Work out the finished part from the listing and answer in its coordinate system (mm). Face numbers are marked on the shaded views. A direction names the side the tool comes from. Round coordinates to 2 decimals unless told otherwise and drop trailing zeros. Order: outer loops, then holes, each group sorted by start corner. A loop starts at its lowest first (then second) coordinate and runs counter-clockwise, first axis right, second up. Notation, with made-up numbers: (-36.5, 58.25) -> (19.5, 58.25) arc R32 cw to (19.5, 89.25) -> close; hole circle Ø5 at (-5, 19). An arc over 180 degrees is marked (long way). Use one line per item in the form item = value.
```python
from build123d import *

# Parameters (mm, degrees)
SALIENTE_EXTRUIR1_DEPTH = 51.5
CORTAR_EXTRUIR2_DEPTH   = 25.75
CROQUIS5_R              = 4.05
CROQUIS5_R_2            = 1.6
CORTAR_EXTRUIR3_DEPTH   = 108.820452605
REDONDEO1_R             = 10
REDONDEO2_R             = 2
REDONDEO3_R             = 2


with BuildPart() as part:
    # Croquis1 → Saliente-Extruir1 (new body)
    with BuildSketch(Plane(origin=(0, 0, 0), x_dir=(1, 0, 0), z_dir=(0, 1, 0))):
        with BuildLine():
            Line((75, -12.5), (-58.334166688, -12.5))
            ThreePointArc((-58.334166688, -12.5), (-61.46808254, -13.003760143), (-64.286250013, -14.464285714))
            ThreePointArc((-64.286250013, -14.464285714), (-93, 0), (-64.286250013, 14.464285714))
            ThreePointArc((-64.286250013, 14.464285714), (-61.46808254, 13.003760143), (-58.334166688, 12.5))
            Line((-58.334166688, 12.5), (75, 12.5))
            ThreePointArc((75, 12.5), (87.5, 0), (75, -12.5))
        make_face()
    extrude(amount=SALIENTE_EXTRUIR1_DEPTH)

    # Croquis3 → Cortar-Extruir2 (cut, symmetric)
    with BuildSketch(Plane.XY):
        Polygon((87.5, 25), (-5, 25), (-31.5, 51.5), (87.5, 51.5), align=None)
        Polygon((-15.355339059, 0), (-41.855339059, 26.5), (-93, 26.5), (-93, 0), align=None)
    extrude(amount=CORTAR_EXTRUIR2_DEPTH, both=True, mode=Mode.SUBTRACT)

    # Croquis4 → Cortar-Revoluci_n1 (revolve, cut)
    with BuildSketch(Plane.XY, mode=Mode.PRIVATE) as cortar_revoluci_n1_sk:
        Polygon((-75, 26.5), (-75, 51.5), (-85, 51.5), (-85, 42.5), (-91.1, 35.5), (-91.1, 26.5), align=None)
    revolve(cortar_revoluci_n1_sk.sketch.rotate(Axis((-75, 26.5, 0), (0, 1, 0)), 270), axis=Axis((-75, 26.5, 0), (0, 1, 0)), mode=Mode.SUBTRACT)

    # Croquis5 → Cortar-Extruir3 (cut, through all)
    with BuildSketch(Plane(origin=(0, 0, 0), x_dir=(1, 0, 0), z_dir=(0, 1, 0))):
        with Locations((75, 0)):
            Circle(CROQUIS5_R)
        with Locations((50, 0)):
            Circle(CROQUIS5_R_2)
    extrude(amount=CORTAR_EXTRUIR3_DEPTH, mode=Mode.SUBTRACT)

    # Redondeo1
    redondeo1_edges = [part.edges().sort_by_distance(p)[0] for p in [
        (-31.5, 51.5, 0),
        (-5, 25, 0),
    ]]
    fillet(redondeo1_edges, radius=REDONDEO1_R)

    # Redondeo2
    redondeo2_edges = [part.edges().sort_by_distance(p)[0] for p in [
        (-61.46808254, 51.5, -13.003760143),
        (-93, 51.5, 0),
        (-61.46808254, 51.5, 13.003760143),
        (-46.988151156, 51.5, 12.5),
        (37.071067812, 25, 12.5),
        (87.5, 25, 0),
        (-18.25, 38.25, 12.5),
        (-18.25, 38.25, -12.5),
        (-31.8153013, 50.738795325, 12.5),
        (-46.988151156, 51.5, -12.5),
        (37.071067812, 25, -12.5),
        (-31.8153013, 50.738795325, -12.5),
        (-4.6846987, 25.761204675, 12.5),
        (-4.6846987, 25.761204675, -12.5),
    ]]
    fillet(redondeo2_edges, radius=REDONDEO2_R)

    # Redondeo3
    redondeo3_edges = [part.edges().sort_by_distance(p)[0] for p in [
        (29.82233047, 0, 12.5),
        (-28.605339059, 13.25, -12.5),
        (-28.605339059, 13.25, 12.5),
        (29.82233047, 0, -12.5),
        (87.5, 0, 0),
    ]]
    fillet(redondeo3_edges, radius=REDONDEO3_R)


solid = part.part
```
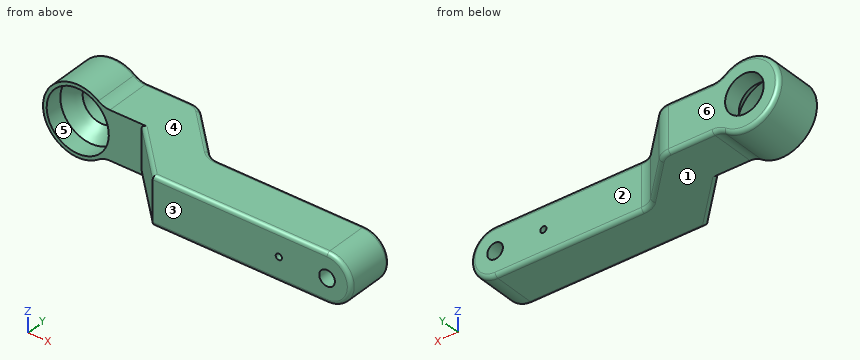
Item 1: The part is cut by section C-C, the plane x = -56.5. Give the vertices of the cut face in (y, z), and give its area (3 significant figures).
Findings:
outline = (26.5, -12.5) -> (49.5, -12.5) arc R2 ccw to (51.5, -10.5) -> (51.5, 10.5) arc R2 ccw to (49.5, 12.5) -> (26.5, 12.5) -> close
area = 623 mm^2
Item 2: Consider line 1 along Z through (x, y) = (50, 18); line 2 along X through (y, z) = (12.75, 0); line 3 along Z through (x, y) = (-75, 29). Determine where each line is inside the solid, lowest interval first.
Findings:
line_1 = -12.5 to -1.6, 1.6 to 12.5
line_2 = -28.11 to 48.4, 51.6 to 70.95, 79.05 to 87.5
line_3 = -18 to -16.1, 16.1 to 18
Item 3: The part is cut by section A-A, the plane x = 50. Give the vertices of the cut face in (y, z), and give its area (3 significant figures).
Findings:
outline = (0, -10.5) arc R2 ccw to (2, -12.5) -> (23, -12.5) arc R2 ccw to (25, -10.5) -> (25, -1.6) -> (0, -1.6) -> close; (0, 1.6) -> (25, 1.6) -> (25, 10.5) arc R2 ccw to (23, 12.5) -> (2, 12.5) arc R2 ccw to (0, 10.5) -> close
area = 542 mm^2
Item 4: The part is cut by section B-B, the plane z = 0. Give the number of separate pieces and of enclosed holes in the cut face, and give its area (3 significant figures).
Findings:
separate_pieces = 4
enclosed_holes = 0
area = 3,850 mm^2
Item 5: Determine the mould class of the marked faces 4, 5 and 6 for opening direction Z: released by +Z, released by -Z, zero draft, split by the parting line, or undercut.
Findings:
face_4 = released by +Z
face_5 = undercut
face_6 = zero draft
Item 6: Flat-ended cylindrical pins translate along their axes: P1, Ø24, axis at x = -16, y = 16, coming from the +Z side; P2, Ø1, axis at x = -60, z = 1, coming from the -Y side; P3, Ø12, axis at x = -48.5, z = -3, coming from the -Y side. Find the tip coordinate at first contact, or state that the pin passes through.
Findings:
P1 = 12.5
P2 = 36.15
P3 = 26.5
Item 7: For the marked faces 1, 2 and 3, determine the directions among +Z, -Z, +X, -X, +Y, -Y from which every point of the face is accessible in a straight line to the end or side of a thin tool.
Findings:
face_1 = -Z, +X, +Y, -Y
face_2 = +Z, -Z, +X, +Y
face_3 = +Z, -Z, +X, -X, -Y
